from build123d import *

# Parameters (mm, degrees)
SKETCH1_W           = 155
SKETCH1_H           = 155
BOSS_EXTRUDE1_DEPTH = 14
SKETCH2_W           = 131.5
SKETCH2_H           = 131.5
SKETCH2_W_2         = 126.5
SKETCH2_H_2         = 126.5
CUT_EXTRUDE1_DEPTH  = 5
SKETCH3_W           = 122.5
SKETCH3_H           = 122.5
CUT_EXTRUDE2_DEPTH  = 111.492081164
SKETCH6_R           = 2.5
CUT_EXTRUDE5_DEPTH  = 11
SKETCH7_R           = 2.5
CUT_EXTRUDE6_DEPTH  = 111.492081164
SKETCH8_W           = 75
SKETCH8_H           = 14
CUT_EXTRUDE7_DEPTH  = 13.25
CUT_EXTRUDE8_START  = -5
SKETCH9_R           = 1
CUT_EXTRUDE8_DEPTH  = 5
FILLET1_R           = 3
SKETCH10_R          = 2.5
CUT_EXTRUDE9_DEPTH  = 10
BOSS_EXTRUDE2_DEPTH = 75
SKETCH11_R          = 63.5
CUT_EXTRUDE10_DEPTH = 111.492081234
FILLET2_R           = 0.5


with BuildPart() as part:
    # Sketch1 → Boss-Extrude1 (new body)
    with BuildSketch(Plane(origin=(0, 0, 0), x_dir=(1, 0, 0), z_dir=(0, 1, 0))):
        Rectangle(SKETCH1_W, SKETCH1_H)
    extrude(amount=BOSS_EXTRUDE1_DEPTH)

    # Sketch2 → Cut-Extrude1 (cut)
    with BuildSketch(Plane(origin=(0, 14, 0), x_dir=(1, 0, 0), z_dir=(0, 1, 0))):
        Rectangle(SKETCH2_W, SKETCH2_H)
        Rectangle(SKETCH2_W_2, SKETCH2_H_2, mode=Mode.SUBTRACT)
    extrude(amount=-CUT_EXTRUDE1_DEPTH, mode=Mode.SUBTRACT)

    # Sketch3 → Cut-Extrude2 (cut, through all)
    with BuildSketch(Plane(origin=(0, 14, 0), x_dir=(1, 0, 0), z_dir=(0, 1, 0))):
        Rectangle(SKETCH3_W, SKETCH3_H)
    extrude(amount=-CUT_EXTRUDE2_DEPTH, mode=Mode.SUBTRACT)

    # Sketch6 → Cut-Extrude5 (cut)
    with BuildSketch(Plane.XY.offset(77.5)):
        with Locations((67.5, 7)):
            Circle(SKETCH6_R)
        with Locations((-67.5, 7)):
            Circle(SKETCH6_R)
    extrude(amount=-CUT_EXTRUDE5_DEPTH, mode=Mode.SUBTRACT)

    # Sketch7 → Cut-Extrude6 (cut, through all)
    with BuildSketch(Plane.XZ):
        with Locations(Location((70, -60.5, 0), (0, 0, 270))):
            Circle(SKETCH7_R)
        with Locations(Location((70, 60.5, 0), (0, 0, 270))):
            Circle(SKETCH7_R)
        with Locations(Location((-70, 60.5, 0), (0, 0, 270))):
            Circle(SKETCH7_R)
        with Locations(Location((-70, -60.5, 0), (0, 0, 270))):
            Circle(SKETCH7_R)
    extrude(amount=-CUT_EXTRUDE6_DEPTH, mode=Mode.SUBTRACT)

    # Sketch8 → Cut-Extrude7 (cut)
    with BuildSketch(Plane.XY.offset(77.5)):
        with Locations((0, 7)):
            Rectangle(SKETCH8_W, SKETCH8_H)
    extrude(amount=-CUT_EXTRUDE7_DEPTH, mode=Mode.SUBTRACT)

    # Sketch9 → Cut-Extrude8 (cut)
    with BuildSketch(Plane(origin=(0, 14, 0), x_dir=(1, 0, 0), z_dir=(0, 1, 0)).offset(CUT_EXTRUDE8_START)):
        with Locations((-65.75, 65.75)):
            Circle(SKETCH9_R)
        with Locations((65.75, 65.75)):
            Circle(SKETCH9_R)
        with Locations((65.75, -65.75)):
            Circle(SKETCH9_R)
        with Locations((-65.75, -65.75)):
            Circle(SKETCH9_R)
    extrude(amount=CUT_EXTRUDE8_DEPTH, mode=Mode.SUBTRACT)

    # Fillet1
    fillet1_edges = [part.edges().sort_by_distance(p)[0] for p in [
        (-64.75, 11.5, 65.75),
        (-65.75, 11.5, 64.75),
        (64.75, 11.5, 65.75),
        (65.75, 11.5, 64.75),
        (64.75, 11.5, -65.75),
        (65.75, 11.5, -64.75),
        (-65.75, 11.5, -64.75),
        (-64.75, 11.5, -65.75),
        (-63.25, 11.5, -63.25),
        (63.25, 11.5, -63.25),
        (63.25, 11.5, 63.25),
        (-63.25, 11.5, 63.25),
    ]]
    fillet(fillet1_edges, radius=FILLET1_R)

    # Sketch10 → Cut-Extrude9 (cut)
    with BuildSketch(Plane(origin=(77.5, 0, 0), x_dir=(0, 0, -1), z_dir=(1, 0, 0))):
        with Locations((50, 7)):
            Circle(SKETCH10_R)
        with Locations((-50, 7)):
            Circle(SKETCH10_R)
    extrude(amount=-CUT_EXTRUDE9_DEPTH, mode=Mode.SUBTRACT)

    # Sketch12 → Boss-Extrude2 (add)
    with BuildSketch(Plane.ZY.offset(-37.5)):
        with BuildLine():
            Line((77.5, 2.5), (77.5, 0))
            Line((77.5, 0), (64.25, 0))
            Line((64.25, 0), (64.25, 9))
            ThreePointArc((64.25, 9), (70.120763928, 4.212518777), (77.5, 2.5))
        make_face()
    extrude(amount=BOSS_EXTRUDE2_DEPTH)

    # Sketch11 → Cut-Extrude10 (cut, through all)
    with BuildSketch(Plane(origin=(0, 14, 0), x_dir=(1, 0, 0), z_dir=(0, 1, 0))):
        Circle(SKETCH11_R)
    extrude(amount=-CUT_EXTRUDE10_DEPTH, mode=Mode.SUBTRACT)

    # Fillet2
    fillet2_edges = [part.edges().sort_by_distance(p)[0] for p in [
        (-63.25, 11.5, 5.629165125),
        (-63.25, 11.5, -5.629165125),
        (-5.629165125, 11.5, -63.25),
        (5.629165125, 11.5, -63.25),
        (63.25, 11.5, -5.629165125),
        (63.25, 11.5, 5.629165125),
        (5.629165125, 11.5, 63.25),
        (-5.629165125, 11.5, 63.25),
    ]]
    fillet(fillet2_edges, radius=FILLET2_R)


solid = part.part
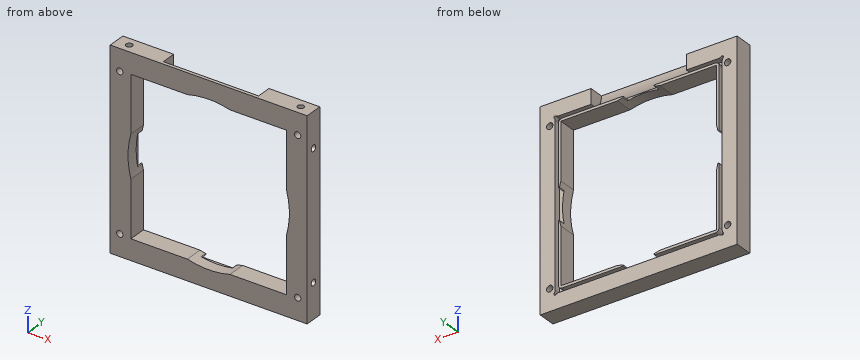
Source: CAD feature listing. Evaluate the final solid. Frame: model axes, mm. Give positions to 0.01 mm unless a question says otherwise; leave off trailing zeros. Write each loop counter-clockwise with the first axis right and the second up, starting at its lowest first coordinate (ties: lowest second). Pieces come first, ordered by that corner, then holes. Notation, with made-up numbers: (46.5, 39) - (98.5, 39) arc R13 cw to (98.5, 48) - close; hole circle Ø9 at (10, -17.5). An arc over 180 degrees is marked (long way). Write item = value, one per line. Start each with the question number.
Q1. Cut plane D-D, the plane y = 7. Give the number of separate pieces and of enclosed holes in the cut face, then the cut area to 3 significant figures.
Q2. Material intervals for probe 1 along X at (y, z) = (3.75, 60.5); probe 2 along X at (y, z) = (10.75, -21); probe 3 along Z at (x, y) = (-37, 1.25), sorted ascending.
Q3. Cut plane B-B, the plane x = -55.5. Return loops of the section in (y, z), then the cut area to 3 significant figures.
Q4. Cut plane A-A, the plane z = -21. Return loops of the section in (x, y), then the cut area to 3 significant figures.
Q5. Pin query (flat end, axial travel): pin 1 Ø1.5 at (y, z) = (6, -50.5) entering from +X; pin 2 Ø1 at (x, y) = (-8.5, 6.5) entering from +Z; pin 3 Ø1.5 at (x, y) = (-28.5, 11.5) entering from +Z. Return the tip coordinate at first contact, or that it passes through.
Q6. Cut plane C-C, the plane z = 50. Return loops of the section in (x, y).
Computed values:
q1.separate_pieces = 1
q1.enclosed_holes = 5
q1.area = 7,670 mm²
q2.probe_1 = -77.5 to -72.5, -67.5 to -61.25, 61.25 to 67.5, 72.5 to 77.5
q2.probe_2 = -77.5 to -65.75, -63.25 to -61.25, 61.25 to 63.25, 65.75 to 77.5
q2.probe_3 = -77.5 to -61.25, 61.25 to 77.5
q3.outline = (0, -77.5) - (14, -77.5) - (14, -65.75) - (9, -65.75) - (9, -63.25) - (14, -63.25) - (14, -61.25) - (0, -61.25) - close; (0, 61.25) - (14, 61.25) - (14, 63.25) - (9, 63.25) - (9, 65.75) - (14, 65.75) - (14, 77.5) - (0, 77.5) - close
q3.area = 430 mm²
q4.outline = (-77.5, 0) - (-61.25, 0) - (-61.25, 14) - (-63.25, 14) - (-63.25, 9) - (-65.75, 9) - (-65.75, 14) - (-77.5, 14) - close; (61.25, 0) - (77.5, 0) - (77.5, 14) - (65.75, 14) - (65.75, 9) - (63.25, 9) - (63.25, 14) - (61.25, 14) - close
q4.area = 430 mm²
q5.pin_1 = 67.5
q5.pin_2 = 67.25
q5.pin_3 = 63.25
q6.outline = (-77.5, 0) - (-61.25, 0) - (-61.25, 14) - (-63.25, 14) - (-63.25, 9) - (-65.75, 9) - (-65.75, 14) - (-77.5, 14) - close; (61.25, 0) - (77.5, 0) - (77.5, 4.5) - (67.5, 4.5) - (67.5, 9.5) - (77.5, 9.5) - (77.5, 14) - (65.75, 14) - (65.75, 9) - (63.25, 9) - (63.25, 14) - (61.25, 14) - close
